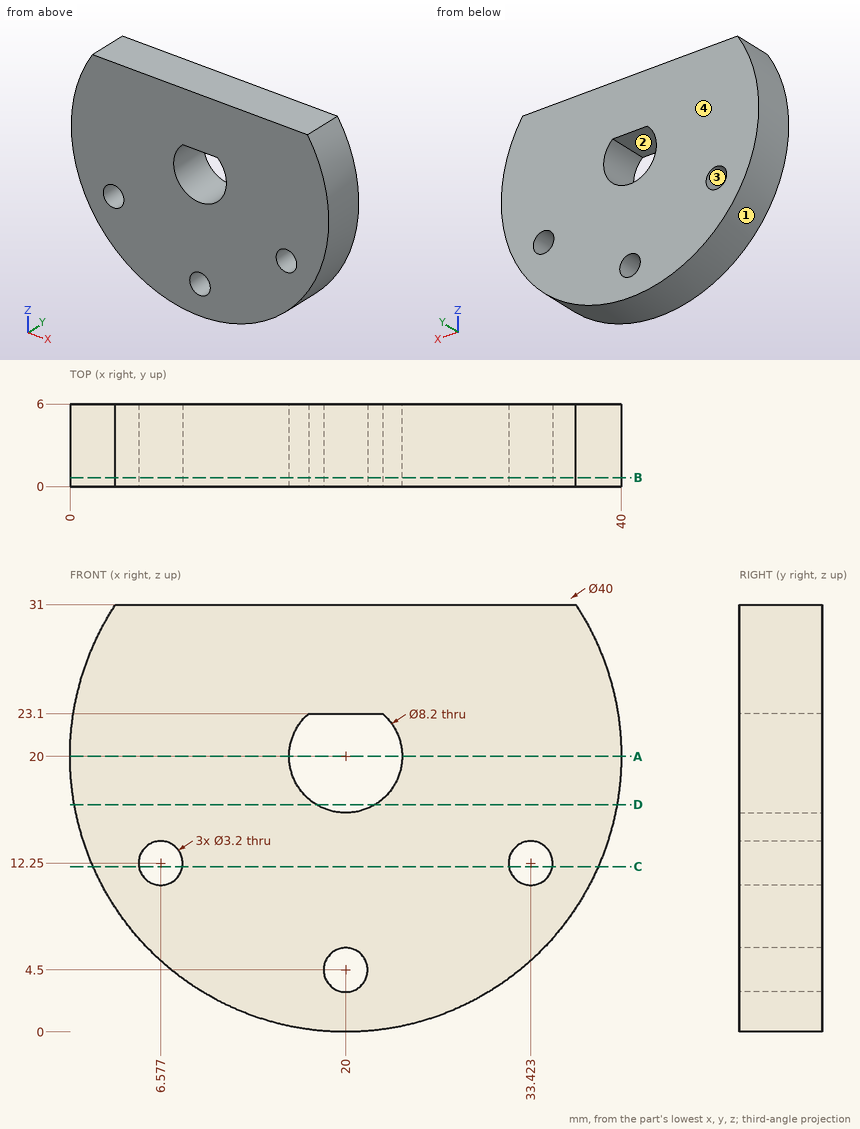
For this review, use the dimensioned drawing (mm, ordinates from the lowest corner) and the shaded views. Coordinates: 2 decimals unless noted, no trailing zeros. Loops run counter-clockwise (first coordinate to the right, second up) from the corner with the lowest first, then second, coordinate; pieces in that order, holes last.
1. Add section B-B, the plane y = 0.65. Give the boundary of the cut face in (x, z), then the cut area to 3 significant figures.
2. Insertion check: P1, Ø12, axis at x = 8, z = 12.5, coming from the +Y side; P2, Ø3, axis at x = 20, z = 4.5, coming from the -Y side. Each pin has a flat end and moves straight along its axis. Give the tip position at first contact, or say it passes through.
3. Mouldability with a two-part tool opening along X and no side actions: class the marked faces 1, 2, 3 and 4 as +X half, -X half, draft (parallel to the pull), parting line (faces both ways), or undercut.
4. Add section A-A, the plane z = 20. Give the boundary of the cut face in (x, y), then the cut area to 3 significant figures.
5. Add section C-C, the plane z = 12. Give the boundary of the cut face in (x, y), then the cut area to 3 significant figures.
6. Add section D-D, the plane z = 16.5. Give the boundary of the cut face in (x, y) (1 decimal), then the cut area to 3 significant figures.
7. For line 1 (Z direction, x = 20, y = 0.5); line 2 (X direction, y = 5.7, z = 9) (1 decimal); line 3 (X direction, y = 4.8, z = 12) (1 decimal), list the stretches that pass through material, from the lowest coordinate up.
Result:
1. outline: (3.3, 31) arc R20 ccw (long way) to (36.7, 31) - close; hole circle Ø3.2 at (6.58, 12.25); hole (17.32, 23.1) arc R4.1 ccw (long way) to (22.68, 23.1) - close; hole circle Ø3.2 at (20, 4.5); hole circle Ø3.2 at (33.42, 12.25)
1. area: 972 mm2
2. P1: stops at y = 6
2. P2: passes through
3. face 1: parting line
3. face 2: undercut
3. face 3: undercut
3. face 4: draft
4. outline: (0, 0) - (15.9, 0) - (15.9, 6) - (0, 6) - close; (24.1, 0) - (40, 0) - (40, 6) - (24.1, 6) - close
4. area: 191 mm2
5. outline: (1.67, 0) - (5, 0) - (5, 6) - (1.67, 6) - close; (8.16, 0) - (31.84, 0) - (31.84, 6) - (8.16, 6) - close; (35, 0) - (38.33, 0) - (38.33, 6) - (35, 6) - close
5. area: 182 mm2
6. outline: (0.3, 0) - (17.9, 0) - (17.9, 6) - (0.3, 6) - close; (22.1, 0) - (39.7, 0) - (39.7, 6) - (22.1, 6) - close
6. area: 211 mm2
7. line 1: z = 0 to 2.9, 6.1 to 15.9, 23.1 to 31
7. line 2: x = 3.3 to 36.7
7. line 3: x = 1.7 to 5, 8.2 to 31.8, 35 to 38.3
